```python
from build123d import *

# Parameters (mm, degrees)
F0_W     = 86
F0_H     = 20
F1_DEPTH = 3
F3_D     = 3
F4_D     = 8
F5_D     = 3


with BuildPart() as f1:
    # F0 (on Top) → F1 (new body)
    with BuildSketch(Plane.XY):
        Rectangle(F0_W, F0_H)
    extrude(amount=F1_DEPTH)

    # F3 (through all)
    with Locations(Plane.XY.offset(3)):
        with Locations((37, 4), (37, -4), (29, -4), (29, 4)):
            Hole(F3_D / 2)

    # F4 (through all)
    with Locations(Plane.XY.offset(3)):
        with Locations((-28, 0)):
            Hole(F4_D / 2)

    # F5 (through all)
    with Locations(Plane.XY.offset(3)):
        with Locations((-34.717514, -6.717514), (-33.656854, 5.656854), (-21.282486, 6.717514), (-22.343146, -5.656854)):
            Hole(F5_D / 2)


solid = f1.part
```
The listing builds one solid part. Answer for the finished solid, in the listing's coordinates (mm). Coordinates: 2 decimals unless noted, no trailing zeros. Order: outer loops, then holes, each group sorted by start corner. A loop starts at its lowest first (then second) coordinate and runs counter-clockwise, first axis right, second up. Notation, with made-up numbers: M 15.5,-0.75 L 44.5,-0.75 A14 ccw 44.5,13.25 Z; hole C -31,60 d4. An arc over 180 degrees is marked long. Answer as a JSON object with one key per item and string values. Group by question number.
1. Determine the mould class of faces 1 (the flat face through (43, 0, 1)), 2 (the cylindrical face through (30.5, 4.07, 1.48)), 3 (the flat face through (-1, -10, 1)) for opening direction Y: released by +Y, released by -Y, zero draft, split by the parting line, or undercut.
2. Section C-C on x = -28 is taken. Write down the section's boundary in (y, z), then the cut area to 3 significant figures.
3. Section D-D on z = 0.55 is taken. State how many separate pieces and enclosed holes the cut face has, then the cut area to 3 significant figures.
4. Section A-A on x = 29 is taken. Write down the section's boundary in (y, z), then the cut area to 3 significant figures.
5. Straight lines are drawn through the part: line 1 (Y direction, x = -21, z = 0.45); line 2 (X direction, y = -3.5, z = 0.1); line 3 (X direction, y = 2.75, z = 2.9). For each, find the intervals that lie inside material, in ascending order.
6. Section B-B on y = 0 is taken. Write down the section's boundary in (x, z).
Values follow:
{
 "1": {"face 1": "zero draft", "face 2": "undercut", "face 3": "released by -Y"},
 "2": {"outline": "M -10,0 L -4,0 L -4,3 L -10,3 Z; M 4,0 L 10,0 L 10,3 L 4,3 Z", "area": "36.0 mm2"},
 "3": {"separate pieces": "1", "enclosed holes": "9", "area": "1,610 mm2"},
 "4": {"outline": "M -10,0 L -5.5,0 L -5.5,3 L -10,3 Z; M -2.5,0 L 2.5,0 L 2.5,3 L -2.5,3 Z; M 5.5,0 L 10,0 L 10,3 L 5.5,3 Z", "area": "42.0 mm2"},
 "5": {"line 1": "-10 to -6.32, -4.99 to 5.24, 8.19 to 10", "line 2": "-43 to -29.94, -26.06 to 27.59, 30.41 to 35.59, 38.41 to 43", "line 3": "-43 to -30.9, -25.1 to 28.17, 29.83 to 36.17, 37.83 to 43"},
 "6": {"outline": "M -43,0 L -32,0 L -32,3 L -43,3 Z; M -24,0 L 43,0 L 43,3 L -24,3 Z"}
}
